```python
from build123d import *

# Parameters (mm, degrees)
BOSS_EXTRUDE1_DEPTH = 10
BOSS_EXTRUDE2_DEPTH = 10
FILLET1_R           = 1
SKETCH4_R           = 2.25
CUT_EXTRUDE1_DEPTH  = 10


with BuildPart() as part:
    # Sketch1 → Boss-Extrude1 (new body)
    with BuildSketch(Plane(origin=(0, 0, 0), x_dir=(1, 0, 0), z_dir=(0, 1, 0))):
        Polygon((0, 0), (2, 0.535898385), (2, 27.5), (0, 27.5), align=None)
    extrude(amount=BOSS_EXTRUDE1_DEPTH)

    # Sketch3 → Boss-Extrude2 (add)
    with BuildSketch(Plane.XZ):
        Polygon((0, 0), (115.911099155, -31.058285412), (115.285791267, -32.958019616), (0, -2), align=None)
    extrude(amount=-BOSS_EXTRUDE2_DEPTH)

    # Fillet1
    fillet1_edges = [part.edges().sort_by_distance(p)[0] for p in [
        (2, 5, -2.537065657),
        (0, 5, 0),
    ]]
    fillet(fillet1_edges, radius=FILLET1_R)

    # Sketch4 → Cut-Extrude1 (cut)
    with BuildSketch(Plane(origin=(-0.500942736, 0, -1.86548043), x_dir=(-0.9657847664118184, 0, 0.25934491505882573), z_dir=(-0.25934491505882573, 0, -0.9657847664118184))):
        with Locations((-8.893504829, 5)):
            Circle(SKETCH4_R)
    extrude(amount=-CUT_EXTRUDE1_DEPTH, mode=Mode.SUBTRACT)


solid = part.part
```
Design review of the part built by this model. Coordinates are the model's own, in mm. A direction names the side the tool comes from. Round coordinates to 2 decimals unless told otherwise and drop trailing zeros. Write each loop counter-clockwise with the first axis right and the second up, starting at its lowest first coordinate (ties: lowest second). Pieces come first, ordered by that corner, then holes.
Item 1: Clearance check with flat-ended pins moving along their axes: pin 1 Ø6 at (x, y) = (59.5, 4.5) entering from -Z; pin 2 Ø3 at (x, y) = (14.5, 7.5) entering from +Z; pin 3 Ø12 at (x, z) = (90.5, -18.5) entering from -Y; pin 4 Ø6 at (x, y) = (69.5, 3.5) entering from -Z. State where each tip first meets the part, or that it passes through.
Item 2: We need section C-C on z = -12. Write out the cut boundary in (x, y).
Item 3: For faces 4 (the flat face through (1, 5, -27.5)), 5 (the flat face through (60.06, 4.93, -18.13)), 6 (the flat face through (115.6, 4.9, -32)), list the 3-axis set-ups (+Z, -Z, +X, -X, +Y, -Y) from which the entire face can be reached by the end or side of a thin tool; tool diameter is ignored.
Item 4: We need section A-A on y = 6. Write out the cut boundary in (x, z).
Item 5: We need section D-D on x = 34. Write out the cut boundary in (y, z), and give its area (3 significant figures).
Item 6: The part is to be moulded in two halves that separate along Y. For faces 1 (the cylindrical face through (7.17, 6.9, -2.94)), 2 (the flat face through (0, 5, -15)), 3 (the flat face through (45, 10, -13)), say which applies: +Y half, -Y half, draft (parallel to the pull), parting line (faces both ways), or undercut.
Item 7: We need section B-B on z = -19. Write out the cut boundary in (x, y), and give its area (3 significant figures).
Item 8: For probe 1 along Z at (x, y) = (63, 0.75); probe 2 along Z at (x, y) = (110, 1.5), list the stretches that pass through material, from the lowest coordinate up.
Returned:
1. pin 1: stops at z = -18.78
1. pin 2: stops at z = -3.48
1. pin 3: stops at y = 0
1. pin 4: stops at z = -21.47
2. outline: (0, 0) - (2, 0) - (2, 10) - (0, 10) - close; (37.24, 0) - (44.78, 0) - (44.78, 10) - (37.24, 10) - close
3. face 4: -Z, -X, +Y, -Y
3. face 5: -Z, +Y, -Y
3. face 6: -Z, +X, +Y, -Y
4. outline: (0, -27.5) - (2, -27.5) - (2, -3.84) arc R1 cw to (3.26, -2.88) - (6.14, -3.65) - (6.64, -1.78) - (1.26, -0.34) arc R1 ccw to (0, -1.3) - close; (10.03, -4.69) - (115.29, -32.96) - (115.91, -31.06) - (10.54, -2.82) - close
5. outline: (0, -11.13) - (10, -11.13) - (10, -9.11) - (0, -9.11) - close
5. area: 20.2 mm2
6. face 1: undercut
6. face 2: draft
6. face 3: +Y half
7. outline: (0, 0) - (2, 0) - (2, 10) - (0, 10) - close; (63.31, 0) - (70.91, 0) - (70.91, 10) - (63.31, 10) - close
7. area: 96.0 mm2
8. probe 1: z = -18.92 to -16.88
8. probe 2: z = -31.54 to -29.47
